```python
from build123d import *

# Parameters (mm, degrees)
SKETCH5_R           = 17.5
BOSS_EXTRUDE1_DEPTH = 5.85
SKETCH8_R           = 4.35
BOSS_EXTRUDE2_DEPTH = 10.25
SKETCH13_R          = 4
SKETCH13_R_2        = 1.35
SKETCH13_R_3        = 3.65
CUT_EXTRUDE1_DEPTH  = 9.55
SKETCH14_R          = 15.5
CUT_EXTRUDE2_DEPTH  = 4.65
SKETCH15_R          = 17.5
BOSS_EXTRUDE3_DEPTH = 2


with BuildPart() as part:
    # Sketch5 → Boss-Extrude1 (new body)
    with BuildSketch(Plane.XY):
        with Locations((70.000455679, -49.499827976)):
            Circle(SKETCH5_R)
    extrude(amount=BOSS_EXTRUDE1_DEPTH)

    # Sketch8 → Boss-Extrude2 (add)
    with BuildSketch(Plane.XY):
        with Locations((79.090811, -46.590809)):
            Circle(SKETCH8_R)
        with Locations((61, -46.5)):
            Circle(SKETCH8_R)
    extrude(amount=BOSS_EXTRUDE2_DEPTH)

    # Sketch13 → Cut-Extrude1 (cut)
    with BuildSketch(Plane.XY):
        with Locations((70.5, -53)):
            Circle(SKETCH13_R)
        with Locations((77, -39.000037614)):
            Circle(SKETCH13_R_2)
        with Locations((62, -58.016959066)):
            Circle(SKETCH13_R_2)
        with Locations((79.090811, -46.590809)):
            Circle(SKETCH13_R_3)
        with Locations((61, -46.5)):
            Circle(SKETCH13_R_3)
    extrude(amount=CUT_EXTRUDE1_DEPTH, mode=Mode.SUBTRACT)

    # Sketch14 → Cut-Extrude2 (cut)
    with BuildSketch(Plane.XY):
        with Locations((70.000455679, -49.499827976)):
            Circle(SKETCH14_R)
    extrude(amount=CUT_EXTRUDE2_DEPTH, mode=Mode.SUBTRACT)

    # Sketch15 → Boss-Extrude3 (add)
    with BuildSketch(Plane(origin=(0, 0, 0), x_dir=(1, 0, 0), z_dir=(0, 0, -1))):
        with Locations((70.000455679, 49.499827976)):
            Circle(SKETCH15_R)
        with BuildLine():
            ThreePointArc((85.500455679, 49.499827976), (82.293609036, 40.059045139), (74.000019478, 34.524732336))
            ThreePointArc((74.000019478, 34.524732336), (70.000004184, 33.999827982), (66.000019478, 34.524965365))
            ThreePointArc((66.000019478, 34.524965365), (60.560030931, 61.793256324), (85.500455679, 49.499827976))
        make_face(mode=Mode.SUBTRACT)
    extrude(amount=BOSS_EXTRUDE3_DEPTH)


solid = part.part
```
Input: part model. Units: mm. Frame: model coordinates. A direction names the side the tool comes from. Give positions to 0.01 mm unless a question says otherwise; leave off trailing zeros. Order: outer loops, then holes, each group sorted by start corner. A loop starts at its lowest first (then second) coordinate and runs counter-clockwise, first axis right, second up. Notation, with made-up numbers: (77.5, 73.25) - (108.5, 73.25) arc R24 cw to (108.5, 107.25) - close; hole circle Ø5 at (-32.5, 38.5). An arc over 180 degrees is marked (long way). Use a Markdown table: item, result.
(1) Access query for faces 1 (the cylindrical face through (57.794, -43.56, 8.019)), 2 (the cylindrical face through (78.247, -39.517, 5.242)), 3 (the cylindrical face through (82.57, -45.49, 7.07)). Directions: +Z, -Z, +X, -X, +Y, -Y. A direction counts if a zero-diameter tool reaches every point of the face in a straight line with its end or side. Return the directions, or none.
Computed values:
| item | result |
|---|---|
| face 1 | +Z |
| face 2 | +Z, -Z |
| face 3 | -Z |
(2) Pin query (flat end, axial travel): pin 1 (5 mm diameter, centred on x = 78, z = 3, fed in from +Y); pin 2 (1 mm diameter, centred on x = 74.5, y = -47, fed in from -Z); pin 3 (5 mm diameter, centred on y = -37.5, z = 1.5, fed in from +X). Return the tip coordinate at first contact, or that it passes through.
Computed values:
| item | result |
|---|---|
| pin 1 | stops at y = -32.89 |
| pin 2 | stops at z = 4.65 |
| pin 3 | stops at x = 84.7 |
(3) Line query: line 1 (Z direction, x = 67.5, y = -64); line 2 (X direction, y = -47.5, z = 7); line 3 (Y direction, x = 72.5, z = -0.25). Output: solid intervals per line, ascending. Write a range as from..to.
Computed values:
| item | result |
|---|---|
| line 1 | z = 4.65..5.85 |
| line 2 | x = 56.77..57.49, 64.51..65.23, 74.84..75.56, 82.63..83.34 |
| line 3 | y = -66.82..-64.8, -34.2..-32.18 |
(4) Section query A-A (x = 70.5). Output: boundary loops of the cut face in (y, z).
Computed values:
| item | result |
|---|---|
| outline | (-66.99, -2) - (-64.99, -2) - (-64.99, 4.65) - (-57, 4.65) - (-57, 5.85) - (-66.99, 5.85) - close; (-49, 4.65) - (-34.01, 4.65) - (-34.01, -2) - (-32.01, -2) - (-32.01, 5.85) - (-49, 5.85) - close |
(5) Draft query along X for faces 4 (the flat face through (79, -47, 10.25)), 5 (the cylindrical face through (72.346, -56.549, 5.242)), 6 (the cylindrical face through (66.207, -32.416, 1.98)). Return one class per face: released by +X, released by -X, zero draft, split by the parting line, or undercut.
Computed values:
| item | result |
|---|---|
| face 4 | zero draft |
| face 5 | undercut |
| face 6 | split by the parting line |
(6) Section query B-B (y = -53). Output: boundary loops of the cut face in (x, z).
Computed values:
| item | result |
|---|---|
| outline | (52.85, -2) - (54.9, -2) - (54.9, 4.65) - (66.5, 4.65) - (66.5, 5.85) - (52.85, 5.85) - close; (74.5, 4.65) - (85.1, 4.65) - (85.1, -2) - (87.15, -2) - (87.15, 5.85) - (74.5, 5.85) - close |
(7) Section query D-D (y = -61). Output: boundary loops of the cut face in (x, z), then the cut area to 3 significant figures.
Computed values:
| item | result |
|---|---|
| outline | (56.81, -2) - (59.61, -2) - (59.61, 4.65) - (80.39, 4.65) - (80.39, -2) - (83.19, -2) - (83.19, 5.85) - (56.81, 5.85) - close |
| area | 68.9 mm2 |
(8) Section query C-C (x = 60). Output: boundary loops of the cut face in (y, z).
Computed values:
| item | result |
|---|---|
| outline | (-63.86, -2) - (-61.34, -2) - (-61.34, 4.65) - (-50.01, 4.65) - (-50.01, 9.55) - (-42.99, 9.55) - (-42.99, 4.65) - (-37.66, 4.65) - (-37.66, -2) - (-35.14, -2) - (-35.14, 5.85) - (-42.27, 5.85) - (-42.27, 10.25) - (-50.73, 10.25) - (-50.73, 5.85) - (-63.86, 5.85) - close |
